Autodesk Fusion 360 part; units mm, degrees
sketch "Sketch1" plane through (0, 0, 0) normal (0, 1, 0) x (1, 0, 0)
  line L0 (47.5, -22.5) -> (-47.5, -22.5)
  line L1 (-47.5, -22.5) -> (-47.5, 22.5)
  line L2 (-47.5, 22.5) -> (47.5, 22.5)
  line L3 (47.5, 22.5) -> (47.5, -22.5)
  line L4 (47.5, -22.5) -> (-47.5, 22.5) construction
  line L5 (-47.5, -22.5) -> (47.5, 22.5) construction
  line L6 (20, -20) -> (-20, -20)
  line L7 (-20, -20) -> (-20, 20)
  line L8 (-20, 20) -> (20, 20)
  line L9 (20, 20) -> (20, -20)
  line L10 (20, -20) -> (-20, 20) construction
  line L11 (-20, -20) -> (20, 20) construction
  circle A0 centre (0, 0) radius 30
  point P0 (-41, 0)
  point P1 (41, 0)
  dimension "d1" = 95
  dimension "d2" = 45
  dimension "d3" = 82
  dimension "d4" = 41
  dimension "d11" = 40
  dimension "d12" = 40
  dimension "d26" = 60
extrude "Extrude1" add sketch "Sketch1" against normal blind 6 contours L0 A0 | L0 L2 A0 | L2 A0 | L6 L7 L8 L9
hole "Hole1" at (-41, 0, 0) at (41, 0, 0) direction (0, -1, 0) diameter 3.4 depth 35 tip angle 118 counterbore diameter 6.5 counterbore depth 3
extrude "Extrude2" add sketch "Sketch1" along normal blind 40 contours L6 L7 L8 L9
sketch "Sketch2" plane through (0, 0, 20) normal (0, 0, 1) x (1, 0, 0)
  line L0 (-20, 0) -> (20, 0)
  line L1 (20, 0) -> (20, 40)
  line L2 (20, 40) -> (-20, 40)
  line L3 (-20, 40) -> (-20, 0)
  point P0 (-10, 30)
  point P1 (10, 30)
  point P2 (10, 10)
  point P3 (-10, 10)
hole "Hole2" at (10, 30, 20) at (-10, 30, 20) at (-10, 10, 20) at (10, 10, 20) direction (0, 0, -1) diameter 3.4 depth 44 tip angle 118
sketch "Sketch3" plane through (0, 40, 0) normal (0, 1, 0) x (-1, 0, 0)
  line L0 (-20, -20) -> (20, -20)
  line L1 (20, -20) -> (20, 20)
  line L2 (20, 20) -> (-20, 20)
  line L3 (-20, 20) -> (-20, -20)
hole "Hole3" at (0, 40, 0) direction (0, -1, 0) diameter 3.5 depth 50 tip angle 118 counterbore diameter 20 counterbore depth 38
equation "d4 = d3 / 2"
Verification items for the finished model (mm, model axes). A direction names the side the tool comes from. Give positions to 0.01 mm unless a question says otherwise; leave off trailing zeros. Write each loop counter-clockwise with the first axis right and the second up, starting at its lowest first coordinate (ties: lowest second). Pieces come first, ordered by that corner, then holes.
(1) Material ranges on line 1 (Y direction, x = 10, z = 7); line 2 (Z direction, x = 0, y = 16); line 3 (X direction, y = 10, z = 18), recorded low to high.
(2) Mould release check, pull along Z, two halves, no side actions. Record for faces 5 (the face through (0, 2, 2)), 6 (the face through (0, 20, 20)), 7 (the face through (11.66, 10.37, -0.28)): +Z half, -Z half, draft (parallel to the pull), parting line (faces both ways), or undercut.
(3) Cross-section at A-A (y = 30). Enter the section's corners in (x, z), plus the area to 3 significant figures.
(4) Cross-section at B-B (y = 19). Enter the section's corners in (x, z), plus the area to 3 significant figures.
(5) Access from +Z, -Z, +X, -X, +Y, -Y to the whole of each face (thin tool, end or side, straight path). Record for faces 1 (the face through (20, 20, 0)), 2 (the face through (0, 20, -20)), 3 (the face through (-9.915, 20.734, -1.302)), 4 (the face through (-20, 20, 0)).
(6) Cross-section at D-D (x = 17). Enter the section's corners in (y, z), plus the area to 3 significant figures.
(7) Gauge pin test, flat ends, axial feed: pin 1 (4 mm diameter, centred on y = -1, z = -15.5, fed in from -X); pin 2 (1.5 mm diameter, centred on y = 30.5, z = -8, fed in from +X); pin 3 (20 mm diameter, centred on x = 4.5, y = 18.5, fed in from +Z); pin 4 (5 mm diameter, centred on y = 35, z = 23, fed in from -X). Record the tip position at first contact, or that the pin passes through.
(8) Cross-section at C-C (z = -19). Enter the section's corners in (x, y), plus the area to 3 significant figures.
Worked out:
1. line 1: y = -6 to 8.3, 11.7 to 28.3, 31.7 to 40
1. line 2: z = -20 to -10, 10 to 20
1. line 3: x = -20 to -11.7, -8.3 to 8.3, 11.7 to 20
2. face 5: undercut
2. face 6: +Z half
2. face 7: draft
3. outline: (-20, -20) - (-11.7, -20) - (-11.7, 20) - (-20, 20) - close; (-8.3, -20) - (8.3, -20) - (8.3, -5.58) arc R10 cw to (-8.3, -5.58) - close; (-8.3, 5.58) arc R10 cw to (8.3, 5.58) - (8.3, 20) - (-8.3, 20) - close; (11.7, -20) - (20, -20) - (20, 20) - (11.7, 20) - close
3. area: 1,040 mm2
4. outline: (-20, -20) - (20, -20) - (20, 20) - (-20, 20) - close; hole circle Ø20 at (0, 0)
4. area: 1,290 mm2
5. face 1: +Z, -Z, +X, +Y
5. face 2: -Z, +X, -X, +Y
5. face 3: +Y
5. face 4: +Z, -Z, -X, +Y
6. outline: (-6, -24.72) - (0, -24.72) - (0, -20) - (40, -20) - (40, 20) - (0, 20) - (0, 24.72) - (-6, 24.72) - close
6. area: 1,900 mm2
7. pin 1: stops at x = -26.79
7. pin 2: stops at x = 20
7. pin 3: stops at z = 20
7. pin 4: passes through
8. outline: (-23.22, -6) - (23.22, -6) - (23.22, 0) - (20, 0) - (20, 40) - (-20, 40) - (-20, 0) - (-23.22, 0) - close; hole circle Ø3.4 at (-10, 10); hole circle Ø3.4 at (-10, 30); hole circle Ø3.4 at (10, 10); hole circle Ø3.4 at (10, 30)
8. area: 1,840 mm2
